Here's the drawing with two shaded views (mm, measured from the low corner). I have some questions. Coordinates: 2 decimals unless noted, no trailing zeros. Loops run counter-clockwise (first coordinate to the right, second up) from the corner with the lowest first, then second, coordinate; pieces in that order, holes last. Notation, with made-up numbers: (-13, 19.5) -> (30, 19.5) arc R30 ccw to (30, 47.5) -> close; hole circle Ø8 at (-39, 44). An arc over 180 degrees is marked (long way). Use CSV: the item, a comma, the result in double quotes. Start each with the question number.
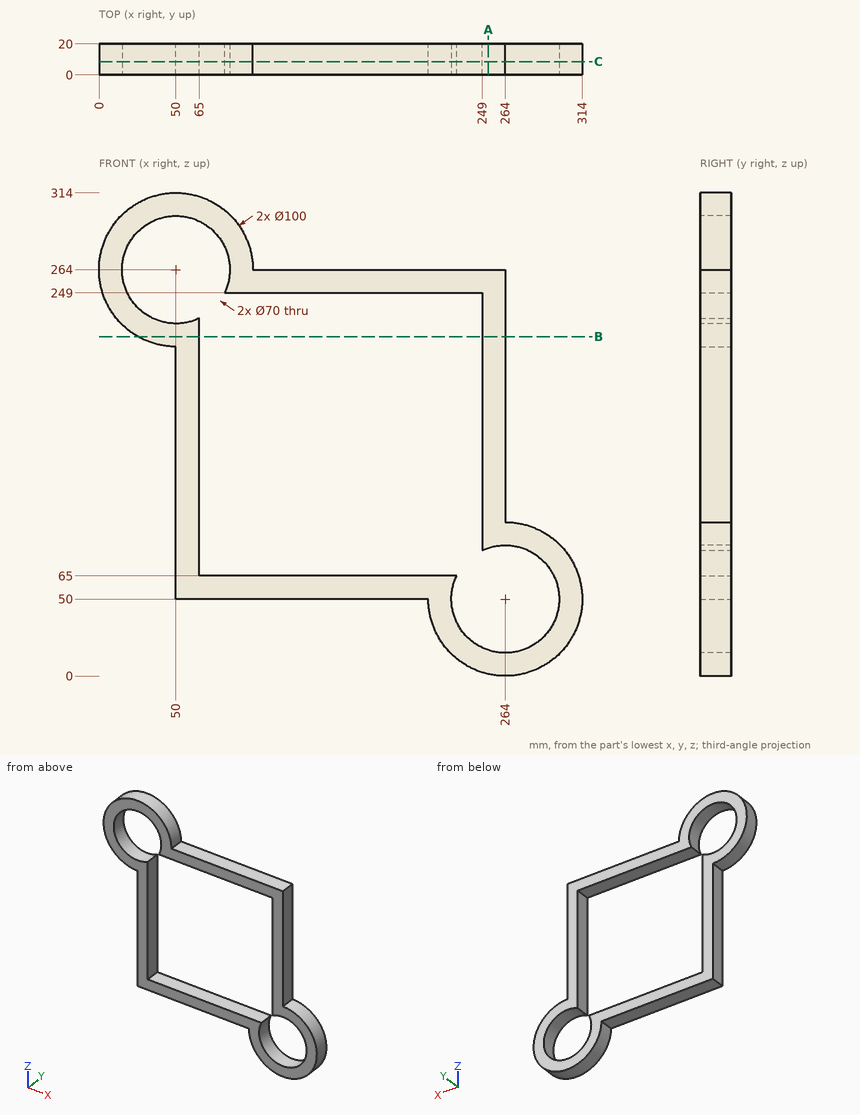
1) I want a section at B-B, the plane z = 220.5. Please give me the cut outline in (x, y), plus the area to 3 significant figures.
2) I want a section at C-C, the plane y = 8.5. Please give me the cut outline in (x, z), plus the area to 3 significant figures.
3) For P1, Ø10, axis at x = 162, y = 8.5, coming from the +Z side; P2, Ø6, axis at x = 141, y = 11, coming from the -Z side; P3, Ø10, axis at y = 5.5, z = 126, coming from the +X side, each with a flat end and sliding along its axis, tell me the tip position at first contact or that it passes through.
4) Please list where these lines run through material, in increasing order: L1, parallel to Z at x = 207, y = 12.75; L2, parallel to X at y = 6.25, z = 31.5. Write a range as [from, to].
5) I want a section at A-A, the plane x = 253. Please give me the cut outline in (y, z) (1 decimal), plus the area to 3 significant figures.
Return value:
1,outline,"(25.35, 0) -> (65, 0) -> (65, 20) -> (25.35, 20) -> close; (249, 0) -> (264, 0) -> (264, 20) -> (249, 20) -> close"
1,area,"1,090 mm²"
2,outline,"(50, 50) -> (214, 50) arc R50 ccw (long way) to (264, 100) -> (264, 264) -> (100, 264) arc R50 ccw (long way) to (50, 214) -> close; hole (65, 65) -> (232.38, 65) arc R35 ccw (long way) to (249, 81.62) -> (249, 249) -> (81.62, 249) arc R35 ccw (long way) to (65, 232.38) -> close"
2,area,"16,400 mm²"
3,P1,"stops at z = 264"
3,P2,"stops at z = 50"
3,P3,"stops at x = 264"
4,L1,"z = [50, 65], [249, 264]"
4,L2,"x = [217.55, 234.29], [293.71, 310.45]"
5,outline,"(0, 1.2) -> (20, 1.2) -> (20, 16.8) -> (0, 16.8) -> close; (0, 83.2) -> (20, 83.2) -> (20, 264) -> (0, 264) -> close"
5,area,"3,930 mm²"
